Autodesk Inventor part; units mm, degrees
ref_plane "YZ Plane" through (0, 0, 0) normal (1, 0, 0) x (0, 1, 0)
ref_plane "XZ Plane" through (0, 0, 0) normal (0, 1, 0) x (-1, 0, 0)
ref_plane "XY Plane" through (0, 0, 0) normal (0, 0, 1) x (1, 0, 0)
ref_plane "Work Plane1" through (0, 0, 0) normal (0, 0, 1) x (1, 0, 0)
sketch "Sketch1" plane through (0, 0, 0) normal (0, 0, 1) x (1, 0, 0)
  line L0 (-30, -73.2876) -> (-18.6416, -61.9292)
  line L1 (-18.6416, -61.9292) -> (-17.5809, -62.9898)
  line L2 (-17.5809, -62.9898) -> (-30, -75.4089)
  line L3 (-30, -75.4089) -> (-30, -76)
  arc A0 (-30, -76) -> (-26, -80) centre (-26, -76) ccw
  line L4 (-18, -80) -> (-26, -80)
  arc A1 (-18, -80) -> (-14, -76) centre (-18, -76) ccw
  line L5 (-14, -34) -> (-14, -76)
  arc A2 (-10, -30) -> (-14, -34) centre (-10, -34) ccw
  line L6 (-10, -30) -> (12, -30)
  arc A3 (16, -34) -> (12, -30) centre (12, -34) ccw
  line L7 (16, -34) -> (16, -76)
  arc A4 (16, -76) -> (20, -80) centre (20, -76) ccw
  line L8 (20, -80) -> (26, -80)
  arc A5 (26, -80) -> (30, -76) centre (26, -76) ccw
  line L9 (30, 28) -> (30, -76)
  line L10 (30, 28) -> (28, 30)
  line L11 (28, 30) -> (-28, 30)
  line L12 (-28, 30) -> (-30, 28)
  line L13 (-30, 28) -> (-30, -73.2876)
  circle A6 centre (-10, -25) radius 1.45
  circle A7 centre (-10, 25) radius 1.45
  circle A8 centre (10, 25) radius 1.45
  circle A9 centre (10, -25) radius 1.45
  circle A10 centre (25, -10) radius 1.45
  circle A11 centre (-25, -10) radius 1.45
  circle A12 centre (-25, 10) radius 1.45
  circle A13 centre (25, 10) radius 1.45
  circle A14 centre (-17.5, -17.5) radius 1.95
  circle A15 centre (17.5, 17.5) radius 1.95
  circle A16 centre (17.5, -17.5) radius 1.95
  circle A17 centre (-17.5, 17.5) radius 1.95
  circle A18 centre (-25, 25) radius 2.325
  circle A19 centre (25, -25) radius 2.325
  circle A20 centre (-25, -25) radius 2.325
  circle A21 centre (25, 25) radius 2.325
  circle A22 centre (0, 0) radius 16
  circle A23 centre (23, -74) radius 3.75
  circle A24 centre (23, -64) radius 1.45
  circle A25 centre (23, -54) radius 1.45
  line L14 (16, -49) -> (46, -49)
  line L15 (46, -49) -> (46, -81)
  line L16 (46, -81) -> (16, -81)
  line L17 (16, -81) -> (16, -49)
  point P0 (0, 0)
  dimension "d0" = 30
  dimension "d1" = 32
  dimension "d2" = 5
extrude "Extrusion1" add sketch "Sketch1" along normal blind 4 contours L14 L15 L16 L17 A4 L8 A5 L9 | L9 A5 L8 A4 L7 L14
sketch "Sketch2" plane through (16, -81, 0) normal (0, -1, 0) x (1, 0, 0)
  line L0 (0, 0) -> (30, 0)
  line L1 (30, 0) -> (30, 4)
  line L2 (0, 4) -> (30, 4)
  line L3 (0, 0) -> (0, 4)
  line L4 (30, 4) -> (26, 4)
  line L5 (26, 4) -> (26, 66)
  line L6 (26, 66) -> (30, 66)
  line L7 (30, 66) -> (30, 4)
  line L8 (30, 66) -> (10, 66)
  line L9 (10, 66) -> (10, 70)
  line L10 (10, 70) -> (30, 70)
  line L11 (30, 70) -> (30, 66)
  point P0 (-16, 0)
  point P1 (26, 4)
  dimension "d5" = 4
  dimension "d6" = 62
  dimension "d7" = 20
  dimension "d8" = 4
extrude "Extrusion2" add sketch "Sketch2" against normal blind 10 contours L2 L5 L6 L7 | L6 L8 L9 L10 L11
fillet "Fillet1" radius 2 4 edges at (46, -76, 70) (42, -76, 4) (44, -71, 4) (46, -65, 0)
sketch "Sketch3" plane through (16, -81, 0) normal (0, -1, 0) x (1, 0, 0)
  line L0 (10, 66) -> (10, 70)
  line L1 (10, 66) -> (12, 66)
  line L2 (12, 66) -> (12, 64)
  line L3 (12, 64) -> (10, 64)
  line L4 (10, 64) -> (10, 66)
  point P0 (-16, 0)
  dimension "d12" = 2
  dimension "d13" = 2
extrude "Extrusion3" add sketch "Sketch3" against normal blind 10
properties part number "30_XY_Sample_lightsheetarm_sample_v3"
Input: part model. Units: mm. Frame: model coordinates. A direction names the side the tool comes from. Round coordinates to 2 decimals unless told otherwise and drop trailing zeros. Order: outer loops, then holes, each group sorted by start corner. A loop starts at its lowest first (then second) coordinate and runs counter-clockwise, first axis right, second up.
1. Cut plane A-A, the plane x = 34.25. Output: boundary loops of the cut face in (y, z), then the cut area to 3 significant figures.
The answers:
outline: (-81, 0) - (-49, 0) - (-49, 4) - (-81, 4) - close; (-81, 66) - (-71, 66) - (-71, 70) - (-81, 70) - close
area: 168 mm2
2. Set-up query: faces 1 (the face through (27, -76, 64)), 2 (the face through (43, -71, 45)), 3 (the face through (31, -65, 4)). Return all of +Z, -Z, +X, -X, +Y, -Y with unobstructed straight access to the full face (end or side cutting, diameter ignored); none if empty.
The answers:
face 1: -X, +Y, -Y
face 2: +Z, +X, -X, +Y
face 3: -X, +Y
3. Cut plane D-D, the plane y = -74. Output: boundary loops of the cut face in (x, z), then the cut area to 3 significant figures.
The answers:
outline: (16, 0) - (19.25, 0) - (19.25, 4) - (16, 4) - close; (26, 64) - (28, 64) - (28, 66) - (42, 66) - (42, 6) arc R2 cw to (40, 4) - (26.75, 4) - (26.75, 0) - (44, 0) arc R2 ccw to (46, 2) - (46, 68) arc R2 ccw to (44, 70) - (26, 70) - close
area: 421 mm2
4. Cut plane B-B, the plane x = 23. Output: boundary loops of the cut face in (y, z), then the cut area to 3 significant figures.
The answers:
outline: (-81, 0) - (-77.75, 0) - (-77.75, 4) - (-81, 4) - close; (-70.25, 0) - (-65.45, 0) - (-65.45, 4) - (-70.25, 4) - close; (-62.55, 0) - (-55.45, 0) - (-55.45, 4) - (-62.55, 4) - close; (-52.55, 0) - (-49, 0) - (-49, 4) - (-52.55, 4) - close
area: 74.8 mm2
5. Cut plane C-C, the plane y = -64. Output: boundary loops of the cut face in (x, z), then the cut area to 3 significant figures.
The answers:
outline: (16, 0) - (21.55, 0) - (21.55, 4) - (16, 4) - close; (24.45, 0) - (44, 0) arc R2 ccw to (46, 2) - (46, 4) - (24.45, 4) - close
area: 108 mm2
6. Mould query, pull axis X, two halves, no side actions, for faces 4 (the face through (35, -76, 66)), 5 (the face through (26, -76, 67)), 6 (the face through (46, -73, 32)). Classes: released by +X, released by -X, zero draft, split by the parting line, or undercut.
The answers:
face 4: undercut
face 5: released by -X
face 6: released by +X
7. Pin query (flat end, axial travel): P1, Ø15, axis at x = 33, y = -61, coming from the +Z side; P2, Ø2, axis at x = 39.5, z = 8, coming from the +Y side; P3, Ø0.6, axis at x = 27, y = -74.5, coming from the -Z side; P4, Ø1.8, axis at y = -78, z = 65.5, coming from the -X side. Return the tip coordinate at first contact, or that it passes through.
The answers:
P1: stops at z = 4
P2: passes through
P3: stops at z = 0
P4: stops at x = 26
8. Material intervals for line 1 (Y direction, x = 23, z = 2.1); line 2 (Z direction, x = 36.5, y = -73); line 3 (Z direction, x = 21.5, y = -59.5), sorted ascending.
The answers:
line 1: y = -81 to -77.75, -70.25 to -65.45, -62.55 to -55.45, -52.55 to -49
line 2: z = 0 to 4, 66 to 70
line 3: z = 0 to 4
